Model file for the job. Use its own axes, mm. Face numbers are marked on the shaded views. A direction names the side the tool comes from. Give positions to 0.01 mm unless a question says otherwise; leave off trailing zeros. Write each loop counter-clockwise with the first axis right and the second up, starting at its lowest first coordinate (ties: lowest second). Pieces come first, ordered by that corner, then holes. Notation, with made-up numbers: (40, 58.25) - (82, 58.25) arc R22 cw to (82, 78.25) - close; hole circle Ø3 at (-34.75, 43). An arc over 180 degrees is marked (long way). Use a Markdown table: item, result. Add a question column.
```python
from build123d import *

# Parameters (mm, degrees)
F0_R     = 7.5
F1_DEPTH = 8.5
F2_R     = 0.5
F3_R     = 7.5
F4_DEPTH = 0.25
F5_R     = 4.75
F6_DEPTH = 1
F7_R     = 1.85
F8_DEPTH = 0.2
F9_R     = 0.25


with BuildPart() as f1:
    # F0 (on Front) → F1 (new body)
    with BuildSketch(Plane.XZ):
        Circle(F0_R)
    extrude(amount=F1_DEPTH)

    # F2
    f2_edges = [f1.edges().sort_by_distance(p)[0] for p in [
        (-7.5, -8.5, 0),
        (-7.5, 0, 0),
    ]]
    fillet(f2_edges, radius=F2_R)

    # F3 (on face) → F4 (join)
    with BuildSketch(Plane.XZ.offset(8.5)):
        Circle(F3_R)
    extrude(amount=F4_DEPTH)

    # F5 (on face) → F6 (join)
    with BuildSketch(Plane.XZ.offset(8.75)):
        Circle(F5_R)
    extrude(amount=F6_DEPTH)

    # F7 (on face) → F8 (join)
    with BuildSketch(Plane.XZ.offset(9.75)):
        Circle(F7_R)
    extrude(amount=F8_DEPTH)

    # F9
    f9_edges = [f1.edges().sort_by_distance(p)[0] for p in [
        (-4.75, -8.75, 0),
        (-4.75, -9.75, 0),
    ]]
    fillet(f9_edges, radius=F9_R)


solid = f1.part
```
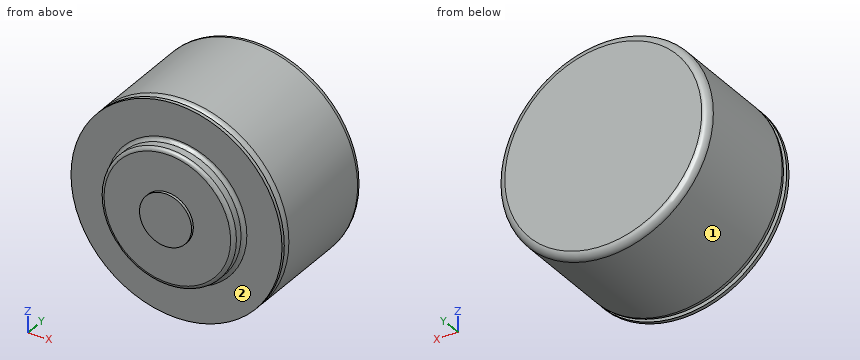
(1) Probe probe 1 along Y at (x, z) = (5, 3.5); probe 2 along Y at (x, z) = (1.75, 3); probe 3 along X at (y, z) = (-2.25, -6). List the from-to ranges inside material, lowest first. Write a range as [from, to].
(2) Which spindle directions (+Z, -Z, +X, -X, +Y, -Y) get a long thin tool onto all of the face, cutting with end or side? Do the marked faces 1 and 2. Say none if no direction does.
(3) Band-saw the part on B-B (z = 0). Write the cut outline in (x, y).
(4) Band-saw the part on A-A (x = 0). Write the cut outline in (y, z), then the cut area to 3 significant figures.
(5) Flat gauge pins, fed straight in: pin 1 (3 mm diameter, centred on y = -5, z = 3, fed in from -X); pin 2 (1.5 mm diameter, centred on x = 6, y = -7.5, fed in from +Z); pin 3 (1.5 mm diameter, centred on x = -4, y = -6, fed in from +Z). Where does each tip first touch, or does it go through?
(6) Band-saw the part on C-C (y = -1.25). Write the cut outline in (x, z), then the cut area to 3 significant figures.
Model answer:
| question | item | result |
|---|---|---|
| 1 | probe 1 | y = [-8.75, 0] |
| 1 | probe 2 | y = [-9.75, 0] |
| 1 | probe 3 | x = [-4.5, 4.5] |
| 2 | face 1 | +Y, -Y |
| 2 | face 2 | -Y |
| 3 | outline | (-7.5, -8.75) - (-5, -8.75) arc R0.25 cw to (-4.75, -9) - (-4.75, -9.5) arc R0.25 ccw to (-4.5, -9.75) - (-1.85, -9.75) - (-1.85, -9.95) - (1.85, -9.95) - (1.85, -9.75) - (4.5, -9.75) arc R0.25 ccw to (4.75, -9.5) - (4.75, -9) arc R0.25 cw to (5, -8.75) - (7.5, -8.75) - (7.5, -8.5) - (7, -8.5) arc R0.5 ccw to (7.5, -8) - (7.5, -0.5) arc R0.5 ccw to (7, 0) - (-7, 0) arc R0.5 ccw to (-7.5, -0.5) - (-7.5, -8) arc R0.5 ccw to (-7, -8.5) - (-7.5, -8.5) - close |
| 4 | outline | (-9.95, -1.85) - (-9.75, -1.85) - (-9.75, -4.5) arc R0.25 ccw to (-9.5, -4.75) - (-9, -4.75) arc R0.25 cw to (-8.75, -5) - (-8.75, -7.5) - (-8.5, -7.5) - (-8.5, -7) arc R0.5 ccw to (-8, -7.5) - (-0.5, -7.5) arc R0.5 ccw to (0, -7) - (0, 7) arc R0.5 ccw to (-0.5, 7.5) - (-8, 7.5) arc R0.5 ccw to (-8.5, 7) - (-8.5, 7.5) - (-8.75, 7.5) - (-8.75, 5) arc R0.25 cw to (-9, 4.75) - (-9.5, 4.75) arc R0.25 ccw to (-9.75, 4.5) - (-9.75, 1.85) - (-9.95, 1.85) - close |
| 4 | area | 141 mm^2 |
| 5 | pin 1 | stops at x = -7.35 |
| 5 | pin 2 | stops at z = 5.36 |
| 5 | pin 3 | stops at z = 6.76 |
| 6 | outline | circle Ø15 at (0, 0) |
| 6 | area | 177 mm^2 |
